The listing builds one solid part. Answer for the finished solid, in the listing's coordinates (mm). Face numbers are marked on the shaded views. A direction names the side the tool comes from. Give positions to 0.01 mm unless a question says otherwise; leave off trailing zeros. Loops run counter-clockwise (first coordinate to the right, second up) from the corner with the lowest first, then second, coordinate; pieces in that order, holes last. Notation, with made-up numbers: (79, 75) - (94, 75) arc R28 cw to (94, 109) - close; hole circle Ø9 at (89, 42.25). An arc over 180 degrees is marked (long way). Answer as CSV lines item,"result". Start each with the question number.
1) A cutting plane is placed at B-B (y = -1.5). Determine the outline of the cut face in (x, z), and give its area (3 significant figures).
2) A cutting plane is placed at D-D (z = -13). Determine the outline of the cut face in (x, y) (3 decimals), and give its area (3 significant figures).
3) A cutting plane is placed at C-C (x = -6). Determine the outline of the cut face in (y, z).
4) A cutting plane is placed at A-A (z = -20). Determine the outline of the cut face in (x, y).
5) For a pull along Z with two mould halves and no side action, classify the marked faces 1, 2 and 3 as pulls with the +Z half, pulls with the -Z half, needs draft (parallel to the pull), parting line crosses it, or undercut.
6) For the marked faces 4, 5 and 6, determine the directions among +Z, -Z, +X, -X, +Y, -Y from which every point of the face is accessible in a straight line to the end or side of a thin tool.
7) Flat-ended cylindrical pins translate along their axes: pin 1 (4 mm diameter, centred on x = -15.5, z = -18.5, fed in from +Y); pin 2 (4 mm diameter, centred on x = 13, y = -6.5, fed in from -Z); pin 3 (5 mm diameter, centred on x = 5.5, z = -41.5, fed in from +Y); pin 4 (6 mm diameter, centred on x = -10, y = 14.5, fed in from +Z). Find the tip coordinate at first contact, or state that the pin passes through.
8) Find the intervals of material crossed by line 1 along Y through (x, z) = (-7.75, -20); line 2 along Y through (x, z) = (13, -11.5); line 3 along Y through (x, z) = (-13, -18), in increasing order.
```python
from build123d import *

# Parameters (mm, degrees)
BOSS_EXTRUDE1_DEPTH     = 61
CUT_EXTRUDE2_DEPTH      = 68.238381896
CUT_EXTRUDE2_DEPTH_BACK = 20
SKETCH3_R               = 9.95
CUT_EXTRUDE3_DEPTH      = 20
CUT_EXTRUDE7_START      = -20
CUT_EXTRUDE7_DEPTH      = 20


# Read off the part's stored shape, not the designer's step: Cut-Extrude7
with BuildPart() as part:
    # Sketch1 → Boss-Extrude1 (new body)
    with BuildSketch(Plane.XY):
        Polygon((0, -10), (20, -10), (20, -20), (-20, -20), (-20, 20), (0, 20), align=None)
    extrude(amount=-BOSS_EXTRUDE1_DEPTH)

    # Sketch2 → Cut-Extrude2 (cut, two sides: drawn at the far end of the back side and taken through both)
    with BuildSketch(Plane(origin=(0, 0, 0), x_dir=(0, 0, -1), z_dir=(1, 0, 0)).offset(-CUT_EXTRUDE2_DEPTH_BACK)):
        with BuildLine():
            Line((0, -138.390030766), (0, 0))
            ThreePointArc((0, 0), (20, 20), (40, 0))
            Line((40, 0), (61, 0))
            Line((61, 0), (199.390030766, 0))
            Line((199.390030766, 0), (41.573756452, 227.379036023))
            Line((41.573756452, 227.379036023), (-157.816274314, 88.989005258))
            Line((-157.816274314, 88.989005258), (0, -138.390030766))
        make_face()
    extrude(amount=CUT_EXTRUDE2_DEPTH + CUT_EXTRUDE2_DEPTH_BACK, mode=Mode.SUBTRACT)

    # Sketch3 → Cut-Extrude3 (cut)
    with BuildSketch(Plane(origin=(0, 0, 0), x_dir=(0, 0, -1), z_dir=(1, 0, 0))):
        with Locations((20, 0)):
            Circle(SKETCH3_R)
    extrude(amount=-CUT_EXTRUDE3_DEPTH, mode=Mode.SUBTRACT)

    # Cut-Extrude7 outline → Cut-Extrude7 (cut)
    with BuildSketch(Plane(origin=(0, 0, 0), x_dir=(0, 0, -1), z_dir=(1, 0, 0)).offset(CUT_EXTRUDE7_START)):
        with BuildLine():
            Line((61, 0), (51, 0))
            ThreePointArc((51, 0), (58.071067812, -2.928932188), (61, -10))
            Line((61, -10), (61, 0))
        make_face()
    extrude(amount=CUT_EXTRUDE7_DEPTH, mode=Mode.SUBTRACT)


solid = part.part
```
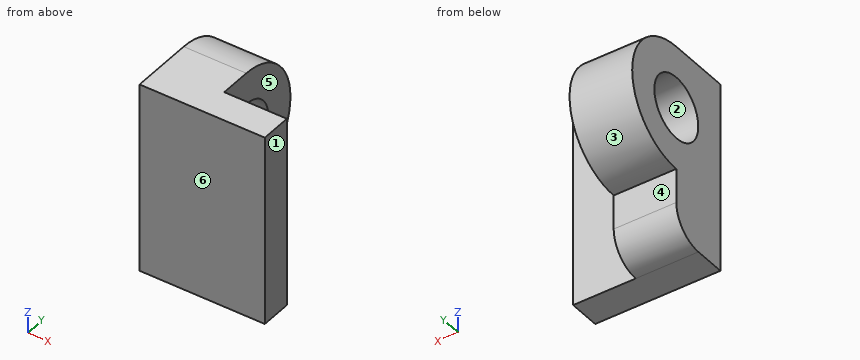
Ans:
1,outline,"(-20, -56.27) - (0, -56.27) - (0, -29.84) - (-20, -29.84) - close; (-20, -10.16) - (0, -10.16) - (0, 0) - (-20, 0) - close"
1,area,"732 mm2"
2,outline,"(-20, -20) - (20, -20) - (20, -10) - (0, -10) - (0, -7.071) - (-20, -7.071) - close; (-20, 7.071) - (0, 7.071) - (0, 18.735) - (-20, 18.735) - close"
2,area,"692 mm2"
3,outline,"(-20, -61) - (-10, -61) arc R10 ccw to (0, -51) - (0, -40) arc R20 ccw to (0, 0) - (-20, 0) - close; hole circle Ø19.9 at (0, -20)"
4,outline,"(-20, -20) - (20, -20) - (20, -10) - (0, -10) - (0, -9.95) - (-20, -9.95) - close; (-20, 9.95) - (0, 9.95) - (0, 20) - (-20, 20) - close"
5,face 1,"needs draft"
5,face 2,"undercut"
5,face 3,"parting line crosses it"
6,face 4,"-Z, +X, -X, +Y"
6,face 5,"+Z, -Z, +X, +Y"
6,face 6,"+Z, -Z, +X, -X, -Y"
7,pin 1,"y = 20"
7,pin 2,"through"
7,pin 3,"y = -10"
7,pin 4,"z = -3.64"
8,line 1,"-20 to -9.95, 9.95 to 20"
8,line 2,"-20 to -10"
8,line 3,"-20 to -9.75, 9.75 to 19.9"
